Print and shaded views of the part. All mm, measured from the part's lowest x, y and z. Coordinates: 2 decimals unless noted, no trailing zeros. Order: outer loops, then holes, each group sorted by start corner. A loop starts at its lowest first (then second) coordinate and runs counter-clockwise, first axis right, second up. Notation, with made-up numbers: (-19.5, -25.5) - (37.5, -25.5) arc R29 cw to (37.5, -5.5) - close; hole circle Ø2 at (81.5, -24). An arc over 180 degrees is marked (long way). Write each question's results on one line, items separated by ' | '.
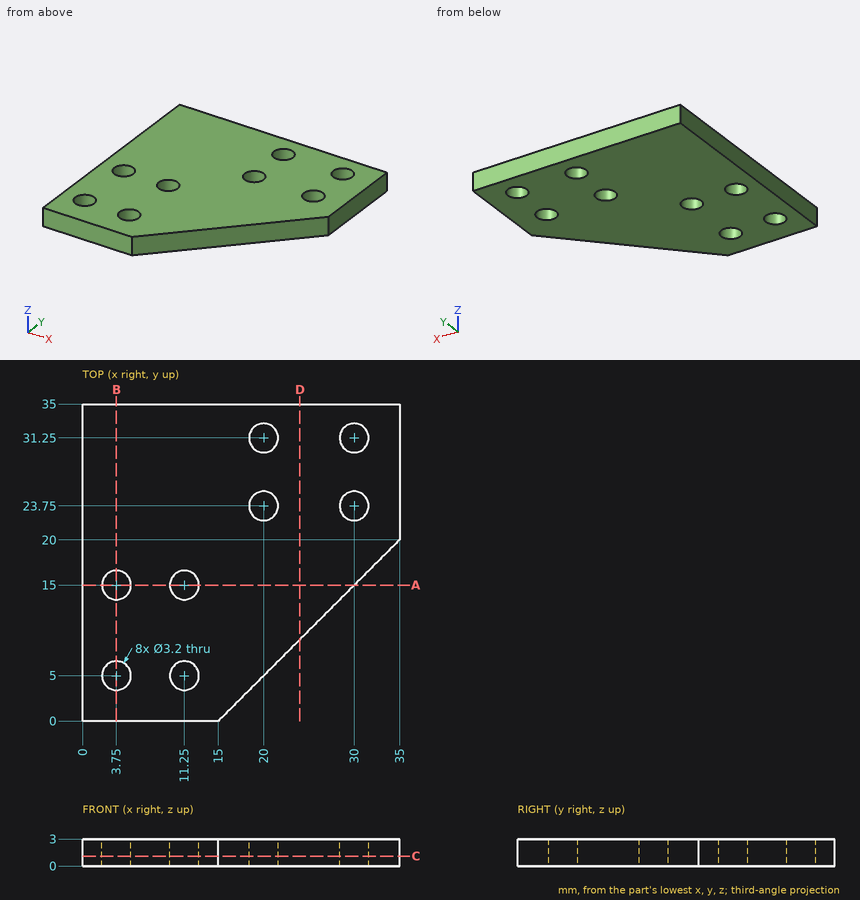
1. Band-saw the part on A-A on y = 15. Give the cut face in (x, z), then the cut area to 3 significant figures.
Solved:
outline: (0, 0) - (2.15, 0) - (2.15, 3) - (0, 3) - close; (5.35, 0) - (9.65, 0) - (9.65, 3) - (5.35, 3) - close; (12.85, 0) - (30, 0) - (30, 3) - (12.85, 3) - close | area: 70.8 mm2
2. Band-saw the part on D-D on x = 24. Give the cut face in (y, z), then the cut area to 3 significant figures.
Solved:
outline: (9, 0) - (35, 0) - (35, 3) - (9, 3) - close | area: 78.0 mm2
3. Band-saw the part on B-B on x = 3.75. Give the cut face in (y, z), then the cut area to 3 significant figures.
Solved:
outline: (0, 0) - (3.4, 0) - (3.4, 3) - (0, 3) - close; (6.6, 0) - (13.4, 0) - (13.4, 3) - (6.6, 3) - close; (16.6, 0) - (35, 0) - (35, 3) - (16.6, 3) - close | area: 85.8 mm2
4. Drop flat-ended pins along their axis: pin 1 Ø2.5 at (x, y) = (20, 31.25) entering from +Z; pin 2 Ø1.5 at (x, z) = (26, 2) entering from -Y. Give the stop position or say it passes through.
Solved:
pin 1: passes through | pin 2: stops at y = 10.25
5. Band-saw the part on C-C on z = 1.1. Give the number of separate pieces and of enclosed holes in the cut face, then the cut area to 3 significant figures.
Solved:
separate pieces: 1 | enclosed holes: 8 | area: 961 mm2
6. Probe line 1 (Y direction, x = 3.75, z = 1.6); line 2 (X direction, y = 14.5, z = 0.15); line 3 (X direction, y = 32, z = 0.8). List the from-to ranges inside material, lowest first.
Solved:
line 1: y = 0 to 3.4, 6.6 to 13.4, 16.6 to 35 | line 2: x = 0 to 2.23, 5.27 to 9.73, 12.77 to 29.5 | line 3: x = 0 to 18.59, 21.41 to 28.59, 31.41 to 35
